Autodesk Inventor part; units mm, degrees
ref_plane "YZ Plane" through (0, 0, 0) normal (1, 0, 0) x (0, 1, 0)
ref_plane "XZ Plane" through (0, 0, 0) normal (0, 1, 0) x (-1, 0, 0)
ref_plane "XY Plane" through (0, 0, 0) normal (0, 0, 1) x (1, 0, 0)
sketch "Sketch1" plane through (0, 0, 0) normal (1, 0, 0) x (0, 1, 0)
  point P0 (0, 0)
sketch "Sketch2" plane through (0, 0, 0) normal (1, 0, 0) x (0, 1, 0)
  line L0 (0, 0) -> (100, 0)
  line L1 (100, 0) -> (100, -300)
  line L2 (100, -300) -> (0, -300)
  line L3 (0, -300) -> (0, 0)
  dimension "d0" = 100
  dimension "d1" = 300
extrude "Extrusion1" add sketch "Sketch2" along normal blind 20
sketch "Sketch3" plane through (20, 0, 0) normal (1, 0, 0) x (0, 0, -1)
  line L0 (0, 0) -> (20, 0)
  line L1 (20, 0) -> (20, 10)
  line L2 (20, 10) -> (0, 10)
  line L3 (0, 0) -> (0, 10)
  line L4 (0, 100) -> (0, 0) construction
  line L5 (0, 20) -> (20, 20)
  line L6 (20, 20) -> (20, 30)
  line L7 (20, 30) -> (0, 30)
  line L8 (0, 20) -> (0, 30)
  line L9 (0, 40) -> (20, 40)
  line L10 (20, 40) -> (20, 50)
  line L11 (20, 50) -> (0, 50)
  line L12 (0, 40) -> (0, 50)
  line L13 (0, 60) -> (20, 60)
  line L14 (20, 60) -> (20, 70)
  line L15 (20, 70) -> (0, 70)
  line L16 (0, 60) -> (0, 70)
  line L17 (0, 80) -> (20, 80)
  line L18 (20, 80) -> (20, 90)
  line L19 (20, 90) -> (0, 90)
  line L20 (0, 80) -> (0, 90)
  line L21 (0, 0) -> (300, 0) construction
  line L22 (280, 0) -> (300, 0)
  line L23 (300, 0) -> (300, 10)
  line L24 (300, 10) -> (280, 10)
  line L25 (280, 0) -> (280, 10)
  line L26 (280, 20) -> (300, 20)
  line L27 (300, 20) -> (300, 30)
  line L28 (280, 20) -> (280, 30)
  line L29 (300, 30) -> (280, 30)
  line L30 (280, 40) -> (300, 40)
  line L31 (300, 40) -> (300, 50)
  line L32 (280, 40) -> (280, 50)
  line L33 (300, 50) -> (280, 50)
  line L34 (280, 60) -> (300, 60)
  line L35 (300, 60) -> (300, 70)
  line L36 (300, 70) -> (280, 70)
  line L37 (280, 80) -> (300, 80)
  line L38 (300, 80) -> (300, 90)
  line L39 (300, 90) -> (280, 90)
  line L40 (280, 80) -> (280, 90)
  line L41 (280, 60) -> (280, 70)
  dimension "d17" = 1
  dimension "d5" = 10
  dimension "d6" = 20
  dimension "d9" = 20
  dimension "d16" = 280
  dimension "d21" = 10
extrude "Extrusion2" cut sketch "Sketch3" against normal blind 64.25
equation "\"d5\" = slot_width"
equation "\"d6\" = pattern_spacing"
equation "\"d9\" = pattern_spacing"
equation "\"d21\" = slot_spacing"
equation "\"slot_spacing\" = 10"
equation "\"slot_width\" = slot_spacing"
equation "\"pattern_spacing\" = 20"
properties part number "Parameter Practice"
Input: part model. Units: mm. Frame: model coordinates. A direction names the side the tool comes from. Give positions to 0.01 mm unless a question says otherwise; leave off trailing zeros. Answer as CSV lines item,"result". Start each with the question number.
1. Line query: L1, parallel to Z at x = 18.5, y = 9.5. Output: solid intervals per line, ascending.
2. Pin query (flat end, axial travel): P1, Ø8, axis at x = 10.5, y = 80.5, coming from the +Z side; P2, Ø3, axis at x = 14, y = 43, coming from the -Z side; P3, Ø1, axis at x = 9.5, y = 26, coming from the +Z side; P4, Ø6, axis at x = 12, z = -285.5, coming from the -Y side. Return the tip coordinate at first contact, or that it passes through.
3. Pull-direction query (Y, two-part tool) for faces 1 (the face through (10, 10, -10)), 2 (the face through (10, 15, 0)), 3 (the face through (10, 20, -290)); classes: released by +Y, released by -Y, zero draft, split by the parting line, or undercut.
4. Reachability of faces 4 (the face through (10, 5, -20)), 5 (the face through (10, 5, -280)), 6 (the face through (10, 90, -10)), 7 (the face through (10, 25, -280)) from +Z, -Z, +X, -X, +Y, -Y: full face, straight path, thin tool, end or side. Return the list, or none.
Computed values:
1,L1,"z = -280 to -20"
2,P1,"stops at z = 0"
2,P2,"stops at z = -280"
2,P3,"stops at z = -20"
2,P4,"stops at y = 10"
3,face 1,"released by -Y"
3,face 2,"zero draft"
3,face 3,"undercut"
4,face 4,"+Z, +X, -X, -Y"
4,face 5,"-Z, +X, -X, -Y"
4,face 6,"+Z, +X, -X"
4,face 7,"-Z, +X, -X"
